```python
from build123d import *

# Parameters (mm, degrees)
SKETCH1_W           = 49
SKETCH1_H           = 49
BOSS_EXTRUDE1_DEPTH = 28.9
SKETCH2_W           = 43
SKETCH2_H           = 43
CUT_EXTRUDE1_DEPTH  = 25.9
CUT_EXTRUDE2_DEPTH  = 46.11884307
CUT_EXTRUDE3_DEPTH  = 15.9


with BuildPart() as part:
    # Sketch1 → Boss-Extrude1 (new body)
    with BuildSketch(Plane.XY):
        Rectangle(SKETCH1_W, SKETCH1_H)
    extrude(amount=BOSS_EXTRUDE1_DEPTH)

    # Sketch2 → Cut-Extrude1 (cut)
    with BuildSketch(Plane(origin=(0, 0, 0), x_dir=(-1, 0, 0), z_dir=(0, 0, -1))):
        Rectangle(SKETCH2_W, SKETCH2_H)
    extrude(amount=-CUT_EXTRUDE1_DEPTH, mode=Mode.SUBTRACT)

    # Sketch3 → Cut-Extrude2 (cut, through all)
    with BuildSketch(Plane.XY.offset(28.9)):
        Polygon((-21.809403406, 8.570892497), (-24.5, 11.26148909), (-24.5, -11.26148909), (-21.809403406, -8.570892497), align=None)
        Polygon((-19.5, -24.5), (-24.5, -19.5), (-24.5, -24.5), align=None)
        Polygon((-9.757939822, -21.943201951), (-11.234107864, -24.5), (11.234107864, -24.5), (9.757939822, -21.943201951), align=None)
        Polygon((24.5, -24.5), (24.5, -19.5), (19.5, -24.5), align=None)
        Polygon((24.5, -11.26148909), (24.5, 11.26148909), (21.809403406, 8.570892497), (21.809403406, -8.570892497), align=None)
        Polygon((-24.5, 19.5), (-19.5, 24.5), (-24.5, 24.5), align=None)
        Polygon((24.5, 24.5), (19.5, 24.5), (24.5, 19.5), align=None)
    extrude(amount=-CUT_EXTRUDE2_DEPTH, mode=Mode.SUBTRACT)

    # Sketch4 → Cut-Extrude3 (cut)
    with BuildSketch(Plane.XY.offset(28.9)):
        with BuildLine():
            Line((-21.809403406, -6.596640664), (-20.73011061, -6.596640664))
            ThreePointArc((-20.73011061, -6.596640664), (-20.151207618, -6.017737672), (-20.73011061, -5.43883468))
            Line((-20.73011061, -5.43883468), (-21.809403406, -5.43883468))
            ThreePointArc((-21.809403406, -5.43883468), (-22.388306399, -6.017737672), (-21.809403406, -6.596640664))
        make_face()
        with BuildLine():
            Line((-21.809403406, -3.596640664), (-20.73011061, -3.596640664))
            ThreePointArc((-20.73011061, -3.596640664), (-20.151207618, -3.017737672), (-20.73011061, -2.43883468))
            Line((-20.73011061, -2.43883468), (-21.809403406, -2.43883468))
            ThreePointArc((-21.809403406, -2.43883468), (-22.388306399, -3.017737672), (-21.809403406, -3.596640664))
        make_face()
        with BuildLine():
            Line((-21.809403406, -0.596640664), (-20.73011061, -0.596640664))
            ThreePointArc((-20.73011061, -0.596640664), (-20.151207618, -0.017737672), (-20.73011061, 0.56116532))
            Line((-20.73011061, 0.56116532), (-21.809403406, 0.56116532))
            ThreePointArc((-21.809403406, 0.56116532), (-22.388306399, -0.017737672), (-21.809403406, -0.596640664))
        make_face()
        with BuildLine():
            Line((-21.809403406, 2.403359336), (-20.73011061, 2.403359336))
            ThreePointArc((-20.73011061, 2.403359336), (-20.151207618, 2.982262328), (-20.73011061, 3.56116532))
            Line((-20.73011061, 3.56116532), (-21.809403406, 3.56116532))
            ThreePointArc((-21.809403406, 3.56116532), (-22.388306399, 2.982262328), (-21.809403406, 2.403359336))
        make_face()
        with BuildLine():
            Line((-21.809403406, 5.403359336), (-20.73011061, 5.403359336))
            ThreePointArc((-20.73011061, 5.403359336), (-20.151207618, 5.982262328), (-20.73011061, 6.56116532))
            Line((-20.73011061, 6.56116532), (-21.809403406, 6.56116532))
            ThreePointArc((-21.809403406, 6.56116532), (-22.388306399, 5.982262328), (-21.809403406, 5.403359336))
        make_face()
        with BuildLine():
            Line((21.809403406, -5.403359336), (20.73011061, -5.403359336))
            ThreePointArc((20.73011061, -5.403359336), (20.151207618, -5.982262328), (20.73011061, -6.56116532))
            Line((20.73011061, -6.56116532), (21.809403406, -6.56116532))
            ThreePointArc((21.809403406, -6.56116532), (22.388306399, -5.982262328), (21.809403406, -5.403359336))
        make_face()
        with BuildLine():
            Line((21.809403406, -2.403359336), (20.73011061, -2.403359336))
            ThreePointArc((20.73011061, -2.403359336), (20.151207618, -2.982262328), (20.73011061, -3.56116532))
            Line((20.73011061, -3.56116532), (21.809403406, -3.56116532))
            ThreePointArc((21.809403406, -3.56116532), (22.388306399, -2.982262328), (21.809403406, -2.403359336))
        make_face()
        with BuildLine():
            Line((21.809403406, 0.596640664), (20.73011061, 0.596640664))
            ThreePointArc((20.73011061, 0.596640664), (20.151207618, 0.017737672), (20.73011061, -0.56116532))
            Line((20.73011061, -0.56116532), (21.809403406, -0.56116532))
            ThreePointArc((21.809403406, -0.56116532), (22.388306399, 0.017737672), (21.809403406, 0.596640664))
        make_face()
        with BuildLine():
            Line((21.809403406, 3.596640664), (20.73011061, 3.596640664))
            ThreePointArc((20.73011061, 3.596640664), (20.151207618, 3.017737672), (20.73011061, 2.43883468))
            Line((20.73011061, 2.43883468), (21.809403406, 2.43883468))
            ThreePointArc((21.809403406, 2.43883468), (22.388306399, 3.017737672), (21.809403406, 3.596640664))
        make_face()
        with BuildLine():
            Line((21.809403406, 6.596640664), (20.73011061, 6.596640664))
            ThreePointArc((20.73011061, 6.596640664), (20.151207618, 6.017737672), (20.73011061, 5.43883468))
            Line((20.73011061, 5.43883468), (21.809403406, 5.43883468))
            ThreePointArc((21.809403406, 5.43883468), (22.388306399, 6.017737672), (21.809403406, 6.596640664))
        make_face()
        with BuildLine():
            Line((5.421097008, -20.863909155), (5.421097008, -21.943201951))
            ThreePointArc((5.421097008, -21.943201951), (6, -22.522104943), (6.578902992, -21.943201951))
            Line((6.578902992, -21.943201951), (6.578902992, -20.863909155))
            ThreePointArc((6.578902992, -20.863909155), (6, -20.285006162), (5.421097008, -20.863909155))
        make_face()
        with BuildLine():
            Line((2.421097008, -20.863909155), (2.421097008, -21.943201951))
            ThreePointArc((2.421097008, -21.943201951), (3, -22.522104943), (3.578902992, -21.943201951))
            Line((3.578902992, -21.943201951), (3.578902992, -20.863909155))
            ThreePointArc((3.578902992, -20.863909155), (3, -20.285006162), (2.421097008, -20.863909155))
        make_face()
        with BuildLine():
            Line((-0.578902992, -20.863909155), (-0.578902992, -21.943201951))
            ThreePointArc((-0.578902992, -21.943201951), (0, -22.522104943), (0.578902992, -21.943201951))
            Line((0.578902992, -21.943201951), (0.578902992, -20.863909155))
            ThreePointArc((0.578902992, -20.863909155), (0, -20.285006162), (-0.578902992, -20.863909155))
        make_face()
        with BuildLine():
            Line((-3.578902992, -20.863909155), (-3.578902992, -21.943201951))
            ThreePointArc((-3.578902992, -21.943201951), (-3, -22.522104943), (-2.421097008, -21.943201951))
            Line((-2.421097008, -21.943201951), (-2.421097008, -20.863909155))
            ThreePointArc((-2.421097008, -20.863909155), (-3, -20.285006162), (-3.578902992, -20.863909155))
        make_face()
        with BuildLine():
            Line((-6.578902992, -20.863909155), (-6.578902992, -21.943201951))
            ThreePointArc((-6.578902992, -21.943201951), (-6, -22.522104943), (-5.421097008, -21.943201951))
            Line((-5.421097008, -21.943201951), (-5.421097008, -20.863909155))
            ThreePointArc((-5.421097008, -20.863909155), (-6, -20.285006162), (-6.578902992, -20.863909155))
        make_face()
    extrude(amount=-CUT_EXTRUDE3_DEPTH, mode=Mode.SUBTRACT)


solid = part.part
```
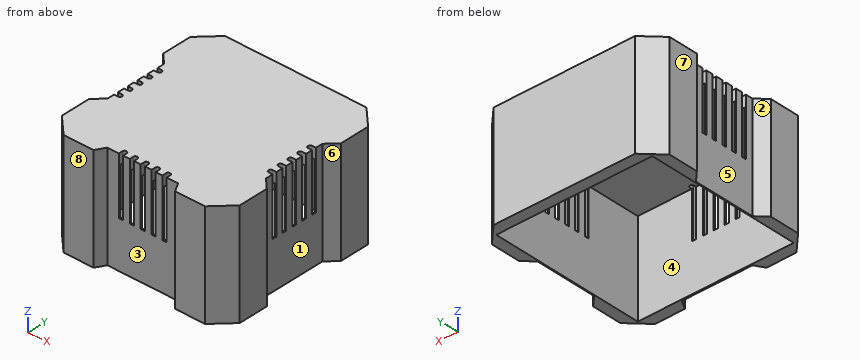
Input: part model. Units: mm. Frame: model coordinates. Face numbers are marked on the shaded views. A direction names the side the tool comes from. Coordinates: 2 decimals unless noted, no trailing zeros. Write each loop counter-clockwise with the first axis right and the second up, starting at its lowest first coordinate (ties: lowest second). Pieces come first, ordered by that corner, then holes.
1) Material intervals for line 1 along Y through (x, z) = (-0.5, 9.5); line 2 along X through (y, z) = (12, 16), sorted ascending.
2) Pin query (flat end, axial travel): pin 1 Ø1.2 at (y, z) = (-21.5, 17.5) entering from -X; pin 2 Ø1 at (y, z) = (7.5, 8) entering from -X; pin 3 Ø3 at (x, y) = (-14.5, 14.5) entering from -Z. Return the tip coordinate at first contact, or that it passes through.
3) Section A-A on z = 4.75. Output: boundary loops of the cut face in (x, y).
4) Section B-B on y = -16. Output: boundary loops of the cut face in (x, z).
5) Mould query, pull axis Y, two halves, no side actions, for the marked faces 5, 6, 7 and 8. Classes: pulls with the +Y half, pulls with the -Y half, needs draft (parallel to the pull), parting line crosses it, or undercut.
6) Set-up query: the marked faces 1, 2, 3 and 4. Return all of +Z, -Z, +X, -X, +Y, -Y with unobstructed straight access to the full face (end or side cutting, diameter ignored); none if empty.
Check result:
1. line 1: y = -21.94 to -21.5, 21.5 to 24.5
1. line 2: x = -24.5 to -21.5, 21.5 to 24.5
2. pin 1: stops at x = -23.1
2. pin 2: stops at x = -21.81
2. pin 3: stops at z = 25.9
3. outline: (-24.5, -19.5) - (-19.5, -24.5) - (-11.23, -24.5) - (-9.76, -21.94) - (9.76, -21.94) - (11.23, -24.5) - (19.5, -24.5) - (24.5, -19.5) - (24.5, -11.26) - (21.81, -8.57) - (21.81, 8.57) - (24.5, 11.26) - (24.5, 19.5) - (19.5, 24.5) - (-19.5, 24.5) - (-24.5, 19.5) - (-24.5, 11.26) - (-21.81, 8.57) - (-21.81, -8.57) - (-24.5, -11.26) - close; hole (-21.5, -21.5) - (21.5, -21.5) - (21.5, 21.5) - (-21.5, 21.5) - close
4. outline: (-24.5, 0) - (-21.5, 0) - (-21.5, 25.9) - (21.5, 25.9) - (21.5, 0) - (24.5, 0) - (24.5, 28.9) - (-24.5, 28.9) - close
5. face 5: undercut
5. face 6: undercut
5. face 7: needs draft
5. face 8: pulls with the -Y half
6. face 1: +Z, -Z, +X
6. face 2: +Z, -Z, -X
6. face 3: +Z, -Z, -Y
6. face 4: -Z
